Check sheet for the drawn part. Datum: minimum x, y, z corner. Units: mm. Coordinates: 2 decimals unless noted, no trailing zeros. Write each loop counter-clockwise with the first axis right and the second up, starting at its lowest first coordinate (ties: lowest second). Pieces come first, ordered by that corner, then holes. Notation, with made-up numbers: M -9.5,81.25 L 24.5,81.25 A7 ccw 24.5,93.25 Z; hole C 41,86.25 d9. An arc over 180 degrees is marked long. Answer in a Markdown table with one row per item.
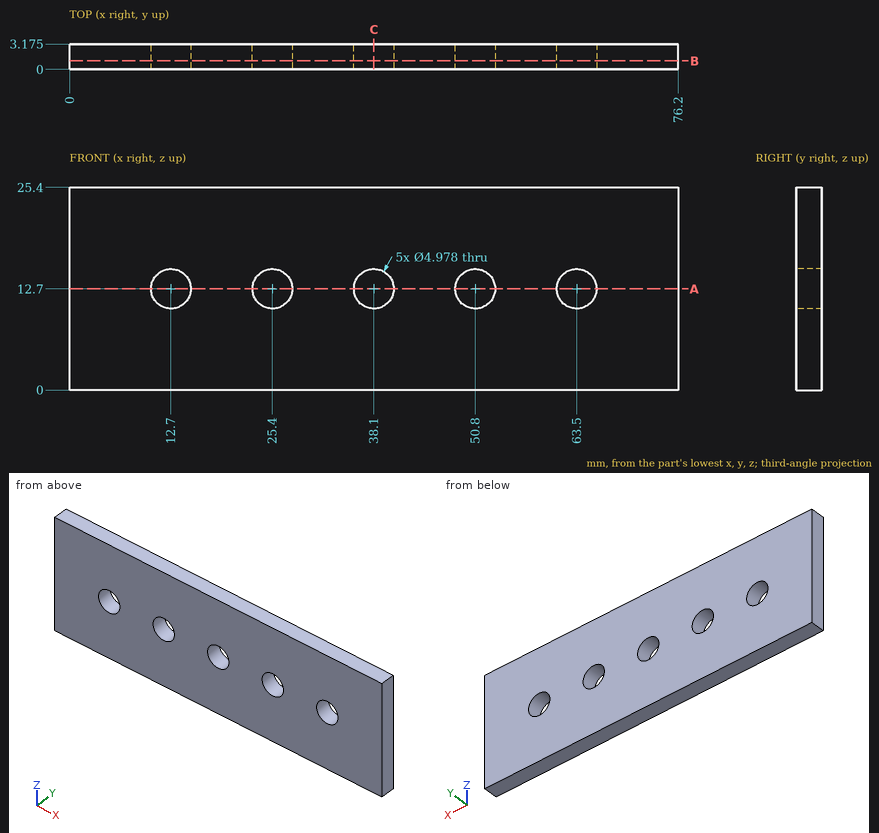
1) Sectioned sample at A-A (z = 12.7). Record the cut outline in (x, y) (1 decimal).
Response values:
| item | result |
|---|---|
| outline | M 0,0 L 10.2,0 L 10.2,3.2 L 0,3.2 Z; M 15.2,0 L 22.9,0 L 22.9,3.2 L 15.2,3.2 Z; M 27.9,0 L 35.6,0 L 35.6,3.2 L 27.9,3.2 Z; M 40.6,0 L 48.3,0 L 48.3,3.2 L 40.6,3.2 Z; M 53.3,0 L 61,0 L 61,3.2 L 53.3,3.2 Z; M 66,0 L 76.2,0 L 76.2,3.2 L 66,3.2 Z |
2) Sectioned sample at C-C (x = 38.1). Record the cut outline in (y, z) (1 decimal).
Response values:
| item | result |
|---|---|
| outline | M 0,0 L 3.2,0 L 3.2,10.2 L 0,10.2 Z; M 0,15.2 L 3.2,15.2 L 3.2,25.4 L 0,25.4 Z |
3) Thickness scan on L1, parallel to X at y = 0.9, z = 12.75; L2, parallel to Z at x = 50.8, y = 2.05; L3, parallel to X at y = 1, z = 13.75. Record the ranges inside material, lowest first. Write a range as [from, to].
Response values:
| item | result |
|---|---|
| L1 | x = [0, 10.21], [15.19, 22.91], [27.89, 35.61], [40.59, 48.31], [53.29, 61.01], [65.99, 76.2] |
| L2 | z = [0, 10.21], [15.19, 25.4] |
| L3 | x = [0, 10.44], [14.96, 23.14], [27.66, 35.84], [40.36, 48.54], [53.06, 61.24], [65.76, 76.2] |
4) Sectioned sample at B-B (y = 1.05). Record the cut outline in (x, z).
Response values:
| item | result |
|---|---|
| outline | M 0,0 L 76.2,0 L 76.2,25.4 L 0,25.4 Z; hole C 12.7,12.7 d4.98; hole C 25.4,12.7 d4.98; hole C 38.1,12.7 d4.98; hole C 50.8,12.7 d4.98; hole C 63.5,12.7 d4.98 |
